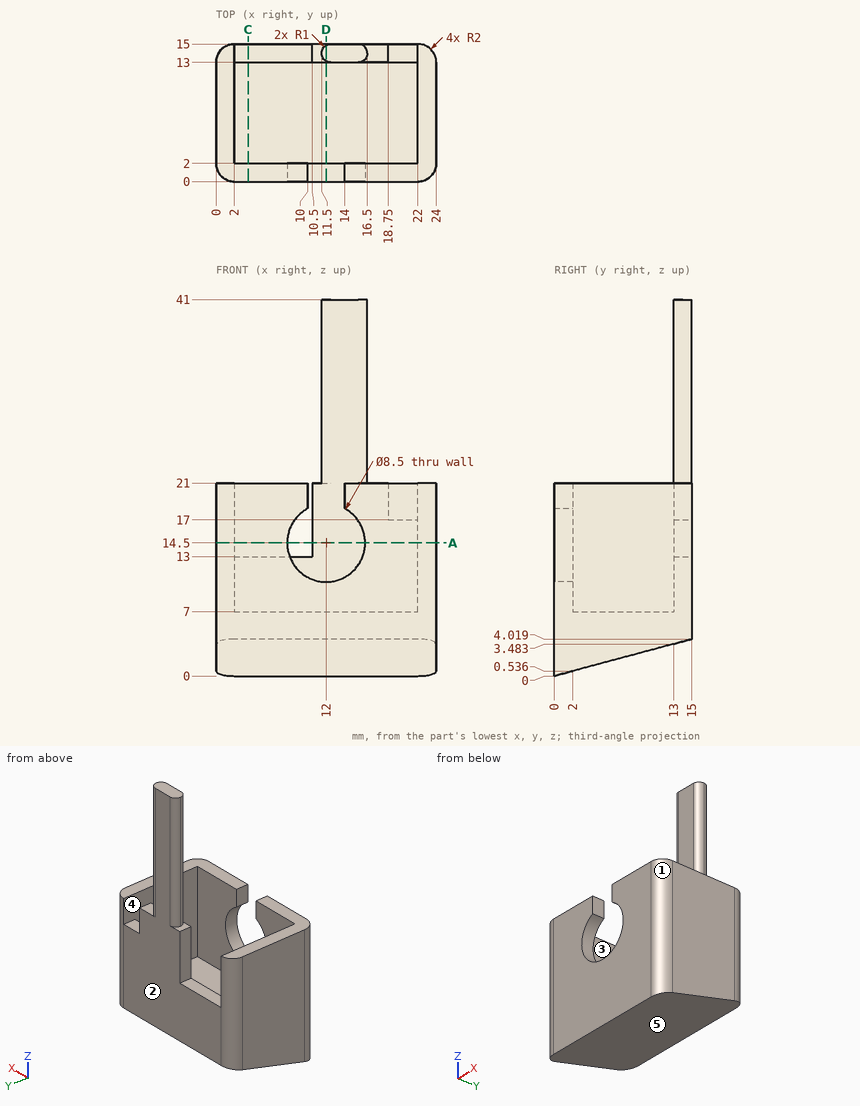
Could you check a few things on this drawing? It's one solid part, dimensions in mm from its lowest x, y, z. A direction names the side the tool comes from. Give positions to 0.01 mm unless a question says otherwise; leave off trailing zeros. Order: outer loops, then holes, each group sorted by start corner. A loop starts at its lowest first (then second) coordinate and runs counter-clockwise, first axis right, second up. Notation, with made-up numbers: M -23,59 L 16,59 A5 cw 16,64 Z; hole C 77.25,69 d3. An arc over 180 degrees is marked long. Use one line per item in the form item = value.
Item 1: Will these pins go through, and if not, where does the flat tip stop? pin 1 Ø2 at (x, y) = (6.5, 3.5) entering from +Z; pin 2 Ø6 at (x, z) = (18.5, 27) entering from -Y; pin 3 Ø0.6 at (y, z) = (14, 20) entering from +X; pin 4 Ø4 at (y, z) = (10.5, 26) entering from -X.
Values follow:
pin_1 = 7
pin_2 = 13
pin_3 = 23.87
pin_4 = through
Item 2: If I drill on line 1 along Y through (x, z) = (11, 11); line 2 along X through (y, z) = (4.25, 8.5); line 3 along Y through (x, z) = (17.75, 16), over which ranges is the centre line in solid material (lowest first)? Write a range as [from, to].
Values follow:
line_1 = [13, 15]
line_2 = [0, 2], [22, 24]
line_3 = [0, 2], [13, 15]
Item 3: Thinking about a two-plate mould opening in Y: for the marked faces 1, 2 and 3, which applies, pulls with the +Y half, pulls with the -Y half, needs draft (parallel to the pull), parting line crosses it, or undercut?
Values follow:
face_1 = pulls with the -Y half
face_2 = pulls with the +Y half
face_3 = undercut
Item 4: For the marked faces 4 and 5, which set-ups out of +Z, -Z, +X, -X, +Y, -Y let a thin tool reach every point of the face, with its end or its side?
Values follow:
face_4 = +Z
face_5 = -Z, +X, -X, +Y
Item 5: If we section it at C-C, the plane x = 3.5: Write out the boundary of the cut face in (y, z), and give its area (3 significant figures).
Values follow:
outline = M 0,0 L 15,4.02 L 15,13 L 13,13 L 13,7 L 2,7 L 2,21 L 0,21 Z
area = 115 mm^2
Item 6: If we section it at A-A, the plane z = 14.5: Write out the boundary of the cut face in (x, y).
Values follow:
outline = M 0,2 A2 ccw 2,0 L 7.75,0 L 7.75,2 L 2,2 L 2,15 A2 ccw 0,13 Z; M 10.5,13 L 22,13 L 22,2 L 16.25,2 L 16.25,0 L 22,0 A2 ccw 24,2 L 24,13 A2 ccw 22,15 L 10.5,15 Z
Item 7: If we section it at D-D, the plane x = 12: Write out the boundary of the cut face in (y, z), and give its area (3 significant figures).
Values follow:
outline = M 0,0 L 15,4.02 L 15,21 L 14.87,21 L 14.87,41 L 13.13,41 L 13.13,21 L 13,21 L 13,7 L 2,7 L 2,10.25 L 0,10.25 Z
area = 144 mm^2
